Geometry: final body of the model. Coordinates: model frame, mm. A direction names the side the tool comes from. Give positions to 0.01 mm unless a question says otherwise; leave off trailing zeros. Write each loop counter-clockwise with the first axis right and the second up, starting at its lowest first coordinate (ties: lowest second). Pieces come first, ordered by that corner, then holes.
Q1. Pin query (flat end, axial travel): pin 1 Ø5 at (x, y) = (-10.5, 6) entering from +Z; pin 2 Ø4 at (x, y) = (-8, 8.5) entering from -Z; pin 3 Ø2 at (x, z) = (-13, -17) entering from +Y. Return the tip coordinate at first contact, or that it passes through.
Q2. Section C-C (z = -15.5). Return the cut outline in (x, y).
Q3. Mould query, pull axis X, two halves, no side actions, for faces 6 (the flat face through (-20, 2, -10)), 7 (the flat face through (-7.25, 8, -14)), 8 (the flat face through (-10, 1, -20)). Classes: +X half, -X half, draft (parallel to the pull), parting line (faces both ways), or undercut.
Q4. Section A-A (x = -11.5). Return the cut outline in (y, z).
Q5. Reachability of faces 1 (the flat face through (-7.25, 8, -6)), 2 (the flat face through (-10, 3, -10)), 3 (the flat face through (-10, 0, -10)), 4 (the flat face through (-10, 3, -18)), 5 (the flat face through (-10, 3, -2)) from +Z, -Z, +X, -X, +Y, -Y: full face, straight path, thin tool, end or side. Return the list, or none.
Q6. Section D-D (x = -5.75). Return the cut outline in (y, z).
Q7. Section B-B (y = 11.5). Return the cut outline in (x, z), plus the area to 3 significant figures.
Q8. Line query: line 1 (Z direction, x = -15, y = 5); line 2 (X direction, y = 8, z = -6); line 3 (Y direction, x = -11.25, z = -2.5). Output: solid intervals per line, ascending.
Autodesk Inventor part; units mm, degrees
ref_plane "YZ Plane" through (0, 0, 0) normal (1, 0, 0) x (0, 1, 0)
ref_plane "XZ Plane" through (0, 0, 0) normal (0, 1, 0) x (-1, 0, 0)
ref_plane "XY Plane" through (0, 0, 0) normal (0, 0, 1) x (1, 0, 0)
sketch "Sketch1" plane through (0, 0, 0) normal (0, 1, 0) x (-1, 0, 0)
  line L0 (0, 0) -> (20, 0)
  line L1 (20, 0) -> (20, -20)
  line L2 (20, -20) -> (0, -20)
  line L3 (0, -20) -> (0, 0)
  dimension "d0" = 20
  dimension "d1" = 20
extrude "Extrusion1" add sketch "Sketch1" along normal blind 3
sketch "Sketch2" plane through (0, 3, 0) normal (0, 1, 0) x (1, 0, 0)
  line L0 (-20, 20) -> (-20, 0)
  line L1 (0, 0) -> (0, 20)
  line L2 (-20, 4.25) -> (0, 4.25)
  line L3 (0, 4.25) -> (0, 7.25)
  line L4 (0, 7.25) -> (-20, 7.25)
  line L5 (-20, 7.25) -> (-20, 4.25)
  line L6 (-20, 15.75) -> (0, 15.75)
  line L7 (0, 15.75) -> (0, 12.75)
  line L8 (0, 12.75) -> (-20, 12.75)
  line L9 (-20, 12.75) -> (-20, 15.75)
  line L10 (0, 20) -> (-20, 20)
  point P0 (0, 15.75)
  point P1 (0, 4.25)
  dimension "d4" = 3
  dimension "d5" = 3
  dimension "d6" = 5.5
  dimension "d7" = 4.25
extrude "Extrusion2" add sketch "Sketch2" along normal blind 10 contours L6 L1 L8 L0 | L4 L1 L2 L0
sketch "Sketch3" plane through (-20, 3, -4.25) normal (0, 0, 1) x (1, 0, 0)
  line L0 (10, 6.25) -> (10, 3.75) construction
  line L1 (0, 10) -> (20, 10)
  line L2 (7.25, 6.25) -> (7.25, 3.75)
  line L3 (12.75, 3.75) -> (12.75, 6.25)
  arc A0 (12.75, 6.25) -> (7.25, 6.25) centre (10, 6.25) ccw
  arc A1 (7.25, 3.75) -> (12.75, 3.75) centre (10, 3.75) ccw
  line L4 (0, 0) -> (0, 10)
  point P0 (20, -3)
  point P1 (10, 5)
  point P2 (10, 1)
  point P3 (10, 9)
  dimension "d10" = 5.5
  dimension "d11" = 10
  dimension "d12" = 8
  dimension "d13" = 9
extrude "Extrusion3" cut sketch "Sketch3" against normal blind 16.75
properties part number "LegStablizer" material "Thermoplastic Resin"
Computed:
1. pin 1: stops at z = -4.25
1. pin 2: stops at z = -15.75
1. pin 3: stops at y = 3
2. outline: (-20, 0) - (0, 0) - (0, 13) - (-20, 13) - close; hole (-12.75, 6.75) arc R2.75 ccw to (-7.25, 6.75) - (-7.25, 9.25) arc R2.75 ccw to (-12.75, 9.25) - close
3. face 6: -X half
3. face 7: undercut
3. face 8: draft
4. outline: (0, -20) - (3, -20) - (3, -15.75) - (4.45, -15.75) - (4.45, -12.75) - (3, -12.75) - (3, -7.25) - (4.45, -7.25) - (4.45, -4.25) - (3, -4.25) - (3, 0) - (0, 0) - close; (11.55, -15.75) - (13, -15.75) - (13, -12.75) - (11.55, -12.75) - close; (11.55, -7.25) - (13, -7.25) - (13, -4.25) - (11.55, -4.25) - close
5. face 1: +Z, -Z
5. face 2: +X, -X, +Y
5. face 3: +Z, -Z, +X, -X, -Y
5. face 4: -Z, +X, -X, +Y
5. face 5: +Z, +X, -X, +Y
6. outline: (0, -20) - (3, -20) - (3, -15.75) - (13, -15.75) - (13, -12.75) - (3, -12.75) - (3, -7.25) - (13, -7.25) - (13, -4.25) - (3, -4.25) - (3, 0) - (0, 0) - close
7. outline: (-20, -15.75) - (-11.58, -15.75) - (-11.58, -12.75) - (-20, -12.75) - close; (-20, -7.25) - (-11.58, -7.25) - (-11.58, -4.25) - (-20, -4.25) - close; (-8.42, -15.75) - (0, -15.75) - (0, -12.75) - (-8.42, -12.75) - close; (-8.42, -7.25) - (0, -7.25) - (0, -4.25) - (-8.42, -4.25) - close
7. area: 101 mm2
8. line 1: z = -15.75 to -12.75, -7.25 to -4.25
8. line 2: x = -20 to -12.75, -7.25 to 0
8. line 3: y = 0 to 3
